```python
from build123d import *

# Parameters (mm, degrees)
BOSS_EXTRUDE1_DEPTH = 7
SKETCH2_R           = 1.25
CUT_EXTRUDE1_DEPTH  = 12
SKETCH3_R           = 6.5
CUT_EXTRUDE2_DEPTH  = 4
SKETCH4_W           = 18
SKETCH4_H           = 7
CUT_EXTRUDE3_DEPTH  = 0.5
CUT_EXTRUDE5_DEPTH  = 10


with BuildPart() as part:
    # Sketch1 → Boss-Extrude1 (new body)
    with BuildSketch(Plane.XY):
        with BuildLine():
            ThreePointArc((18, 18), (9, 27), (0, 18))
            Line((0, 18), (3.5, 18))
            ThreePointArc((3.5, 18), (9, 23.5), (14.5, 18))
            Line((14.5, 18), (18, 18))
        make_face()
        with BuildLine():
            Line((3.5, 18), (0, 18))
            ThreePointArc((0, 18), (9, 9), (18, 18))
            Line((18, 18), (14.5, 18))
            ThreePointArc((14.5, 18), (9, 12.5), (3.5, 18))
        make_face()
        with BuildLine():
            Line((0, 18), (0, 0))
            Line((0, 0), (18, 0))
            Line((18, 0), (18, 18))
            ThreePointArc((18, 18), (9, 9), (0, 18))
        make_face()
    extrude(amount=BOSS_EXTRUDE1_DEPTH)

    # Sketch2 → Cut-Extrude1 (cut)
    with BuildSketch(Plane.XZ):
        with Locations(Location((15, 3.5, 0), (0, 0, 270))):
            Circle(SKETCH2_R)
        with Locations(Location((3, 3.5, 0), (0, 0, 270))):
            Circle(SKETCH2_R)
    extrude(amount=-CUT_EXTRUDE1_DEPTH, mode=Mode.SUBTRACT)

    # Sketch3 → Cut-Extrude2 (cut)
    with BuildSketch(Plane.XY.offset(7)):
        with Locations((9, 18)):
            Circle(SKETCH3_R)
    extrude(amount=-CUT_EXTRUDE2_DEPTH, mode=Mode.SUBTRACT)

    # Sketch4 → Cut-Extrude3 (cut)
    with BuildSketch(Plane.XZ):
        with Locations((9, 3.5)):
            Rectangle(SKETCH4_W, SKETCH4_H)
    extrude(amount=-CUT_EXTRUDE3_DEPTH, mode=Mode.SUBTRACT)

    # Sketch5 → Cut-Extrude5 (cut)
    with BuildSketch(Plane(origin=(0, 0, 0), x_dir=(-1, 0, 0), z_dir=(0, 0, -1))):
        Polygon((-9, 10.170210674), (-6.004587273, 2.662945465), (-11.995412727, 2.662945465), align=None)
    extrude(amount=-CUT_EXTRUDE5_DEPTH, mode=Mode.SUBTRACT)


solid = part.part
```
Build history of the part. All positions in model axes, mm. A direction names the side the tool comes from. Coordinates: 2 decimals unless noted, no trailing zeros. Order: outer loops, then holes, each group sorted by start corner. A loop starts at its lowest first (then second) coordinate and runs counter-clockwise, first axis right, second up. Notation, with made-up numbers: (85, 22.5) -> (140, 22.5) arc R31 cw to (140, 57.5) -> close; hole circle Ø8 at (-13.5, -24.5). An arc over 180 degrees is marked (long way). Answer in a Markdown table with one row per item. Add a question column.
Q1. Wall check: line 1 along X through (y, z) = (18, 1.3); line 2 along X through (y, z) = (5, 3.5); line 3 along X through (y, z) = (6.25, 3.5). Give the ranges that are in metal, low to high. Write a range as [from, to].
Q2. Band-saw the part on D-D, the plane y = 16.5. List the corners of the cut face in (x, z).
Q3. Mould opens along Z. For faces 1 (the face through (3, 12, 4)), 2 (the face through (4, 21, 3)), 3 (the face through (0, 9, 3)), 4 (the face through (16.054, 6.17, 2.828)) say: +Z half, -Z half, draft (parallel to the pull), parting line (faces both ways), or undercut.
Q4. Band-saw the part on A-A, the plane z = 3.5. List the corners of the cut face in (x, y).
Q5. Drop flat-ended pins along their axis: pin 1 (0.8 mm diameter, centred on x = 15, z = 4, fed in from -Y); pin 2 (6.5 mm diameter, centred on x = 6.5, y = 20, fed in from +Z); pin 3 (2 mm diameter, centred on x = 3, z = 3.5, fed in from +Y). Give the stop position or say it passes through.
Q6. Which spindle directions (+Z, -Z, +X, -X, +Y, -Y) get a long thin tool onto all of the face, cutting with end or side? Do faces 5 (the face through (15, 12, 4)), 6 (the face through (9, 11, 0)), 7 (the face through (9, 0.5, 4)), 8 (the face through (12.494, 23.481, 5.028)), 9 (the face through (7.523, 6.469, 3.451)). Say none if no direction does.
Q7. Band-saw the part on B-B, the plane y = 3.5. List the corners of the cut face in (x, z), then the cut area to 3 significant figures.
Q8. Band-saw the part on C-C, the plane x = 11.25. List the corners of the cut face in (y, z).
Answers follow:
| question | item | result |
|---|---|---|
| 1 | line 1 | [0, 3.5], [14.5, 18] |
| 1 | line 2 | [0, 1.75], [4.25, 6.94], [11.06, 13.75], [16.25, 18] |
| 1 | line 3 | [0, 1.75], [4.25, 7.44], [10.56, 13.75], [16.25, 18] |
| 2 | outline | (0, 0) -> (3.71, 0) -> (3.71, 3) -> (2.68, 3) -> (2.68, 7) -> (0, 7) -> close; (14.29, 0) -> (18, 0) -> (18, 7) -> (15.32, 7) -> (15.32, 3) -> (14.29, 3) -> close |
| 3 | face 1 | undercut |
| 3 | face 2 | +Z half |
| 3 | face 3 | draft |
| 3 | face 4 | undercut |
| 4 | outline | (0, 0.5) -> (1.75, 0.5) -> (1.75, 12) -> (4.25, 12) -> (4.25, 0.5) -> (13.75, 0.5) -> (13.75, 12) -> (16.25, 12) -> (16.25, 0.5) -> (18, 0.5) -> (18, 18) arc R9 ccw to (0, 18) -> close; hole circle Ø13 at (9, 18); hole (6, 2.66) -> (12, 2.66) -> (9, 10.17) -> close |
| 5 | pin 1 | y = 12 |
| 5 | pin 2 | z = 3 |
| 5 | pin 3 | y = 25.48 |
| 6 | face 5 | -Y |
| 6 | face 6 | -Z, +X, -X, +Y, -Y |
| 6 | face 7 | +Z, -Z, +X, -X, -Y |
| 6 | face 8 | +Z |
| 6 | face 9 | +Z, -Z |
| 7 | outline | (0, 0) -> (6.34, 0) -> (6.34, 7) -> (0, 7) -> close; (11.66, 0) -> (18, 0) -> (18, 7) -> (11.66, 7) -> close; hole circle Ø2.5 at (3, 3.5); hole circle Ø2.5 at (15, 3.5) |
| 7 | area | 78.9 mm^2 |
| 8 | outline | (0.5, 0) -> (2.66, 0) -> (2.66, 7) -> (0.5, 7) -> close; (4.53, 0) -> (12.98, 0) -> (12.98, 3) -> (11.9, 3) -> (11.9, 7) -> (4.53, 7) -> close; (23.02, 0) -> (26.71, 0) -> (26.71, 7) -> (24.1, 7) -> (24.1, 3) -> (23.02, 3) -> close |
